The model under review builds one solid part; all positions refer to its coordinate system, in mm. A direction names the side the tool comes from. Round coordinates to 2 decimals unless told otherwise and drop trailing zeros. Order: outer loops, then holes, each group sorted by start corner. A loop starts at its lowest first (then second) coordinate and runs counter-clockwise, first axis right, second up. Notation, with made-up numbers: M 67.25,-20.75 L 102.25,-20.75 A21 cw 102.25,-4.75 Z; hole C 58.5,-38 d11. An arc over 180 degrees is marked long. Use a Markdown table: item, result. Add a question column.
1. The part is to be moulded in two halves that separate along X. For faces 1 (the flat face through (-50, 46, 1)), 2 (the flat face through (-1, 0, -1)), 3 (the flat face through (47.5, 47, 1)), say which applies: +X half, -X half, draft (parallel to the pull), parting line (faces both ways), or undercut.
2. For faces 4 (the flat face through (-15, 60, -44)), 5 (the flat face through (49, 58, -6.5)), 6 (the flat face through (-1, 2.5, -1)), list the 3-axis set-ups (+Z, -Z, +X, -X, +Y, -Y) from which the entire face can be reached by the end or side of a thin tool; tool diameter is ignored.
3. To check wall thickness, follow probe 1 along X at (y, z) = (8, 3); probe 2 along Z at (x, y) = (-3.5, 62.5); probe 3 along Y at (x, z) = (-39, -35.5). State the ranges of each line that lie inside material, in increasing order.
4. Consider section D-D on y = 9. State the section outline as (x, z) points.
5. Consider section C-C on y = 42.5. State the section outline as (x, z) points.
6. Insertion check: P1, Ø8, axis at x = -19.5, y = 65.5, coming from the -Z side; P2, Ø10, axis at x = 3, z = -21, coming from the +Y side. Each pin has a flat end and moves straight along its axis. Give the tip position at first contact, or say it passes through.
7. Consider section B-B on z = -28. State the section outline as (x, y) points.
8. Consider section A-A on x = -14.5. State the section outline as (y, z) points, then the cut area to 4 significant figures.
from build123d import *

# Parameters (mm, degrees)
SKETCH1_W           = 100
SKETCH1_H           = 90
SKETCH1_W_2         = 95
SKETCH1_H_2         = 85
BOSS_EXTRUDE1_DEPTH = 2.5
SKETCH1_3_W         = 100
SKETCH1_3_H         = 90
SKETCH1_3_W_2       = 95
SKETCH1_3_H_2       = 85
BOSS_EXTRUDE2_DEPTH = 93
SKETCH2_W           = 32
SKETCH2_H           = 36
CUT_EXTRUDE1_DEPTH  = 5
SKETCH3_W           = 20
SKETCH3_H           = 10
CUT_EXTRUDE2_DEPTH  = 5


with BuildPart() as part:
    # Sketch1 → Boss-Extrude1 (new body)
    # profile 1 of 2: a face of its own
    with BuildSketch(Plane(origin=(0, 0, 0), x_dir=(1, 0, 0), z_dir=(0, 1, 0))):
        Rectangle(SKETCH1_W, SKETCH1_H)
        Rectangle(SKETCH1_W_2, SKETCH1_H_2, mode=Mode.SUBTRACT)
    # profile 2 of 2: a face of its own
    with BuildSketch(Plane(origin=(0, 0, 0), x_dir=(1, 0, 0), z_dir=(0, 1, 0))):
        Rectangle(SKETCH1_W_2, SKETCH1_H_2)
    extrude(amount=BOSS_EXTRUDE1_DEPTH)

    # Sketch1_3 → Boss-Extrude2 (add)
    with BuildSketch(Plane(origin=(0, 0, 0), x_dir=(1, 0, 0), z_dir=(0, 1, 0))):
        Rectangle(SKETCH1_3_W, SKETCH1_3_H)
        Rectangle(SKETCH1_3_W_2, SKETCH1_3_H_2, mode=Mode.SUBTRACT)
    extrude(amount=BOSS_EXTRUDE2_DEPTH)

    # Sketch2 → Cut-Extrude1 (cut)
    with BuildSketch(Plane(origin=(50, 0, 0), x_dir=(0, 0, -1), z_dir=(1, 0, 0))):
        with Locations((-22.5, 58)):
            Rectangle(SKETCH2_W, SKETCH2_H)
        with BuildLine():
            Line((-23, 81.625), (-22, 81.625))
            ThreePointArc((-22, 81.625), (-20.875, 80.5), (-22, 79.375))
            Line((-22, 79.375), (-23, 79.375))
            ThreePointArc((-23, 79.375), (-24.125, 80.5), (-23, 81.625))
        make_face()
        with BuildLine():
            Line((-23, 34.375), (-22, 34.375))
            ThreePointArc((-22, 34.375), (-20.875, 35.5), (-22, 36.625))
            Line((-22, 36.625), (-23, 36.625))
            ThreePointArc((-23, 36.625), (-24.125, 35.5), (-23, 34.375))
        make_face()
        with Locations((22.5, 58)):
            Rectangle(SKETCH2_W, SKETCH2_H)
        with BuildLine():
            Line((23, 34.375), (22, 34.375))
            ThreePointArc((22, 34.375), (20.875, 35.5), (22, 36.625))
            Line((22, 36.625), (23, 36.625))
            ThreePointArc((23, 36.625), (24.125, 35.5), (23, 34.375))
        make_face()
        with BuildLine():
            Line((23, 81.625), (22, 81.625))
            ThreePointArc((22, 81.625), (20.875, 80.5), (22, 79.375))
            Line((22, 79.375), (23, 79.375))
            ThreePointArc((23, 79.375), (24.125, 80.5), (23, 81.625))
        make_face()
    extrude(amount=-CUT_EXTRUDE1_DEPTH, mode=Mode.SUBTRACT)

    # Sketch3 → Cut-Extrude2 (cut)
    with BuildSketch(Plane(origin=(0, 0, -45), x_dir=(-1, 0, 0), z_dir=(0, 0, -1))):
        with Locations((15, 65)):
            Rectangle(SKETCH3_W, SKETCH3_H)
    extrude(amount=-CUT_EXTRUDE2_DEPTH, mode=Mode.SUBTRACT)


solid = part.part
Answer block:
| question | item | result |
|---|---|---|
| 1 | face 1 | -X half |
| 1 | face 2 | draft |
| 1 | face 3 | undercut |
| 2 | face 4 | -Z |
| 2 | face 5 | +X |
| 2 | face 6 | +Y |
| 3 | probe 1 | -50 to -47.5, 47.5 to 50 |
| 3 | probe 2 | -45 to -42.5, 42.5 to 45 |
| 3 | probe 3 | 0 to 2.5 |
| 4 | outline | M -50,-45 L 50,-45 L 50,45 L -50,45 Z; hole M -47.5,-42.5 L 47.5,-42.5 L 47.5,42.5 L -47.5,42.5 Z |
| 5 | outline | M -50,-45 L 50,-45 L 50,-38.5 L 47.5,-38.5 L 47.5,-42.5 L -47.5,-42.5 L -47.5,42.5 L 47.5,42.5 L 47.5,38.5 L 50,38.5 L 50,45 L -50,45 Z; M 47.5,-6.5 L 50,-6.5 L 50,6.5 L 47.5,6.5 Z |
| 6 | P1 | z = 42.5 |
| 6 | P2 | y = 2.5 |
| 7 | outline | M -50,0 L 50,0 L 50,40 L 47.5,40 L 47.5,2.5 L -47.5,2.5 L -47.5,93 L -50,93 Z; M 47.5,76 L 50,76 L 50,93 L 47.5,93 Z |
| 8 | outline | M 0,-45 L 60,-45 L 60,-42.5 L 2.5,-42.5 L 2.5,42.5 L 93,42.5 L 93,45 L 0,45 Z; M 70,-45 L 93,-45 L 93,-42.5 L 70,-42.5 Z |
| 8 | area | 652.5 mm^2 |
